Here's how the part is built. I have some questions about the finished solid (model axes, mm). Coordinates: 2 decimals unless noted, no trailing zeros. Write each loop counter-clockwise with the first axis right and the second up, starting at its lowest first coordinate (ties: lowest second). Pieces come first, ordered by that corner, then holes. Notation, with made-up numbers: (43, 42.25) -> (78, 42.25) arc R19 cw to (78, 69.25) -> close; hole circle Ø1 at (50.25, 59.25). An arc over 180 degrees is marked (long way). Put each result on its own line as item: value. Start each with the question number.
Item 1: I need wall thicknesses on line 1 (Y direction, x = -151, z = 0.75); line 2 (X direction, y = -156.5, z = 0.75); line 3 (X direction, y = 2.5, z = 1.2). Which ranges of each line are inside material? Lowest first, please. Write a range as [from, to].
Item 2: I want a section at A-A, the plane x = -103. State how many separate pieces and enclosed holes the cut face has, then the cut area to 3 significant figures.
Item 3: I want a section at B-B, the plane y = 92.5. List the corners of the cut face in (x, z) for me.
Item 4: For pin 1 (1 mm diameter, centred on y = -47, z = 1, fed in from +X); pin 2 (1 mm diameter, centred on x = -158, z = 0.5, fed in from +Y); pin 3 (1 mm diameter, centred on y = 108, z = 1, fed in from -X), each with a flat end and sliding along its axis, tell me the tip position at first contact or that it passes through.
from build123d import *

# Parameters (mm, degrees)
BOSS_EXTRUDE1_DEPTH = 2
SKETCH2_W           = 100
SKETCH2_H           = 11.123940721
CUT_EXTRUDE1_DEPTH  = 2
LPATTERN1_COUNT     = 7
LPATTERN1_PITCH     = 50
CUT_EXTRUDE2_REACH  = 249.495
SKETCH4_W           = 15
SKETCH4_H           = 350


with BuildPart() as part:
    # Sketch1 → Boss-Extrude1 (new body)
    with BuildSketch(Plane.XY):
        Polygon((-15, -175), (-15, 175), (-150, 175), (-150, 75), (-175, 75), (-175, -75), (-150, -75), (-150, -175), align=None)
    extrude(amount=BOSS_EXTRUDE1_DEPTH)

    # Sketch2 → Cut-Extrude1 (cut)
    with BuildSketch(Plane.XY.offset(2)):
        with Locations((-80, 154.43802964)):
            Rectangle(SKETCH2_W, SKETCH2_H)
    cut_extrude1 = extrude(amount=-CUT_EXTRUDE1_DEPTH, mode=Mode.SUBTRACT)

    # LPattern1: Cut-Extrude1 ×7
    with Locations(*[(0, -i * LPATTERN1_PITCH, 0) for i in range(1, LPATTERN1_COUNT)]):
        add(cut_extrude1, mode=Mode.SUBTRACT)

    # Sketch4 → Cut-Extrude2 (cut, up to next)
    with BuildSketch(Plane.XY.offset(2), mode=Mode.PRIVATE) as cut_extrude2_sk1:
        with Locations((-22.5, 0)):
            Rectangle(SKETCH4_W, SKETCH4_H)
    cut_extrude2_tool1 = extrude(cut_extrude2_sk1.sketch, amount=-CUT_EXTRUDE2_REACH, mode=Mode.PRIVATE) & part.part
    add(cut_extrude2_tool1.solids().sort_by_distance((-22.5, 0, 2))[0], mode=Mode.SUBTRACT)


solid = part.part
Calculated:
1. line 1: y = [-75, 75]
1. line 2: x = [-150, -30]
1. line 3: x = [-175, -130]
2. separate pieces: 8
2. enclosed holes: 0
2. area: 544 mm2
3. outline: (-150, 0) -> (-30, 0) -> (-30, 2) -> (-150, 2) -> close
4. pin 1: stops at x = -130
4. pin 2: stops at y = 75
4. pin 3: stops at x = -150
